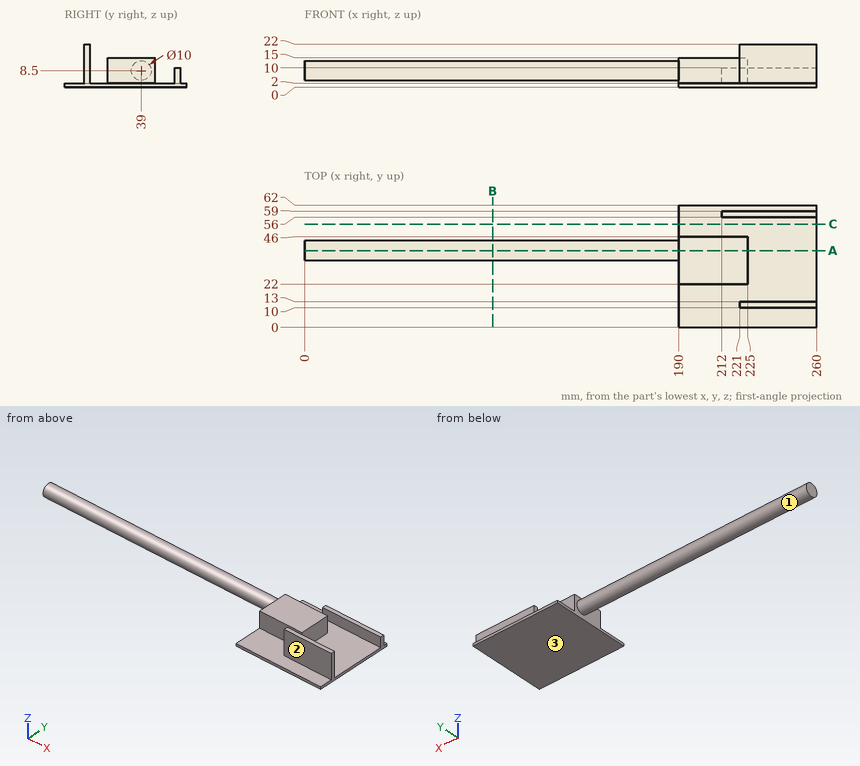
Can you work these out from the drawing? Everything is in mm from the part's minimum corner. A direction names the side the tool comes from. Coordinates: 2 decimals unless noted, no trailing zeros. Loops run counter-clockwise (first coordinate to the right, second up) from the corner with the lowest first, then second, coordinate; pieces in that order, holes last. Notation, with made-up numbers: (-24, 20.25) - (-5, 20.25) arc R28 ccw to (-5, 56.25) - close; hole circle Ø10 at (22.25, 56.5). An arc over 180 degrees is marked (long way). Put each result on its own line as item: value. Start each with the question number.
Item 1: Suppose I cut it at C-C (y = 52.5). Please give me the cut outline in (x, z).
Item 2: Suppose I cut it at B-B (x = 95.5). Please give me the cut outline in (y, z).
Item 3: If I drill on line 1 along Z through (x, y) = (213.5, 27); line 2 along X through (y, z) = (42.5, 3); line 3 along Z through (x, y) = (198.5, 18.5), over which ranges is the centre line in solid material (lowest first)?
Item 4: Suppose I cut it at A-A (y = 39). Please give me the cut outline in (x, z), and give its area (4 significant figures).
Item 5: Which directions (+Z, -Z, +X, -X, +Y, -Y) give clear straight access to the entire face, cutting with the end or side of a thin tool? Please do the marked faces 1, 2 and 3.
Item 6: For pin 1 (2.5 mm diameter, centred on x = 233, z = 6, fed in from -Y); pin 2 (10 mm diameter, centred on x = 223, y = 33.5, fed in from +Z); pin 3 (2.5 mm diameter, centred on x = 235.5, y = 57, fed in from +Z); pin 4 (5 mm diameter, centred on x = 66.5, z = 17.5, fed in from +Y), each with a flat end and sliding along its axis, tell me the tip position at first contact or that it passes through.
Here are the results:
1. outline: (190, 0) - (260, 0) - (260, 2) - (190, 2) - close
2. outline: circle Ø10 at (39, 8.5)
3. line 1: 0 to 15
3. line 2: 190 to 225
3. line 3: 0 to 2
4. outline: (0, 3.5) - (190, 3.5) - (190, 0) - (260, 0) - (260, 2) - (225, 2) - (225, 15) - (190, 15) - (190, 13.5) - (0, 13.5) - close
4. area: 2,495 mm²
5. face 1: -X
5. face 2: +Z, +X, -X, -Y
5. face 3: -Z, +X, -X, +Y, -Y
6. pin 1: y = 10
6. pin 2: z = 15
6. pin 3: z = 10
6. pin 4: through
